Can you work these out from the model? Positions are in its coordinate system, mm. A direction names the side the tool comes from. Give positions to 0.01 mm unless a question says otherwise; leave off trailing zeros. Loops run counter-clockwise (first coordinate to the right, second up) from the corner with the lowest first, then second, coordinate; pieces in that order, holes last. Notation, with made-up numbers: (69.25, 76.25) - (96.25, 76.25) arc R35 cw to (96.25, 113.25) - close; hole circle Ø3 at (70, 32). An arc over 180 degrees is marked (long way). Answer as a JSON object with one key per item and string values. Group by question number.
Item 1: Suppose I cut it at B-B on z = 734.5. Write out the boundary of the cut face in (x, y), and give its area (3 significant figures).
Item 2: Suppose I cut it at C-C on x = -270. Write out the boundary of the cut face in (y, z), and give its area (3 significant figures).
Item 3: Suppose I cut it at D-D on x = -35. Write out the boundary of the cut face in (y, z), and give its area (3 significant figures).
Item 4: Suppose I cut it at A-A on y = 309.5. Write out the boundary of the cut face in (x, z).
Item 5: Which directions (+Z, -Z, +X, -X, +Y, -Y) give clear straight access to the entire face, cutting with the end or side of a thin tool? Please do faces 1 (the flat face through (-19, 461, 1160)), 2 (the flat face through (-7, 520, 1158.4)), 3 (the flat face through (-105.32, 697.036, 1159.211)).
Item 6: Will these pins go through, and if not, where does the flat tip stop? pin 1 (0.8 mm diameter, centred on x = -33.5, z = 0.5, fed in from +Y); pin 2 (10 mm diameter, centred on x = -288.5, z = 500.5, fed in from -Y); pin 3 (1.8 mm diameter, centred on x = 0.5, z = 512, fed in from +Y).
Item 7: Thinking about a two-plate mould opening in Y: for faces 4 (the flat face through (1.6, 236, 572)), 5 (the flat face through (-7, 517, 1.6)), 6 (the flat face through (-262, 801.6, 572)), 7 (the flat face through (-25, 0, 572)), which applies, pulls with the +Y half, pulls with the -Y half, needs draft (parallel to the pull), parting line crosses it, or undercut?
Item 8: Please list where these lines run through material, in increasing order: L1, parallel to Z at x = -15, y = 622; L2, parallel to Y at x = -251, z = 136; L3, parallel to X at y = 584, z = 485.
Autodesk Inventor part; units mm, degrees
ref_plane "YZ Plane" through (0, 0, 0) normal (1, 0, 0) x (0, 1, 0)
ref_plane "XZ Plane" through (0, 0, 0) normal (0, 1, 0) x (-1, 0, 0)
ref_plane "XY Plane" through (0, 0, 0) normal (0, 0, 1) x (1, 0, 0)
sketch "Sketch1" plane through (0, 0, 0) normal (0, 0, 1) x (1, 0, 0)
  line L0 (-347.6, 800) -> (-180, 800)
  line L1 (-180, 800) -> (0, 620)
  line L2 (-180, 800) -> (122.4624, 800) construction
  line L3 (0, 0) -> (0, 620)
  line L4 (0, 0) -> (-50, 0)
  line L5 (-50, -1.6) -> (1.6, -1.6)
  line L6 (1.6, -1.6) -> (1.6, 620.6627)
  line L7 (1.6, 620.6627) -> (-179.3373, 801.6)
  line L8 (-179.3373, 801.6) -> (-347.6, 801.6)
  line L9 (-347.6, 801.6) -> (-347.6, 800)
  line L10 (-50, 0) -> (-50, -1.6)
  dimension "d0" = 167.6
  dimension "d1" = 45
  dimension "d2" = 800
  dimension "d4" = 50
  dimension "d15" = 180
  dimension "d19" = 1.6
extrude "Extrusion1" add sketch "Sketch1" along normal blind 1160
sketch "Sketch2" plane through (0, 0, 0) normal (-1, 0, 0) x (0, 0, -1)
  line L0 (-195, -320) -> (-845, -320) construction
  line L1 (-845, -245) -> (-195, -245)
  line L2 (-195, -245) -> (-195, -395)
  line L3 (-195, -395) -> (-845, -395)
  line L4 (-845, -395) -> (-845, -245)
  point P0 (0, 0)
  dimension "d8" = 195
  dimension "d10" = 650
  dimension "d11" = 650
  dimension "d12" = 150
  dimension "d20" = 320
extrude "Extrusion3" cut sketch "Sketch2" against normal through all
sketch "Sketch3" plane through (0, 0, 0) normal (0, 0, -1) x (-1, 0, 0)
  line L0 (50, 0) -> (0, 0)
  line L1 (0, 0) -> (0, 620)
  line L2 (0, 620) -> (180, 800)
  line L3 (180, 800) -> (347.6, 800)
  line L4 (347.6, 780) -> (188.2843, 780)
  line L5 (188.2843, 780) -> (20, 611.7157)
  line L6 (20, 611.7157) -> (20, 20)
  line L7 (20, 20) -> (50, 20)
  line L8 (347.6, 780) -> (347.6, 800)
  line L9 (50, 20) -> (50, 0)
  dimension "d23" = 20
extrude "Extrusion4" add sketch "Sketch3" against normal blind 1.6
sketch "Sketch4" plane through (0, 0, 1160) normal (0, 0, 1) x (1, 0, 0)
  line L0 (0, 0) -> (-50, 0)
  line L1 (0, 620) -> (0, 0)
  line L2 (-180, 800) -> (0, 620)
  line L3 (-347.6, 800) -> (-180, 800)
  line L4 (-347.6, 800) -> (-347.6, 780)
  line L5 (-347.6, 780) -> (-188.2843, 780)
  line L6 (-188.2843, 780) -> (-20, 611.7157)
  line L7 (-20, 611.7157) -> (-20, 20)
  line L8 (-20, 20) -> (-50, 20)
  line L9 (-50, 20) -> (-50, 0)
extrude "Extrusion5" add sketch "Sketch4" against normal blind 1.6
sketch "Sketch5" plane through (-347.6, 801.6, 0) normal (-1, 0, 0) x (0, 0, 1)
  line L0 (1.6, -1.6) -> (1.6, -21.6)
  line L1 (1.6, -1.6) -> (1158.4, -1.6)
  line L2 (1158.4, -21.6) -> (1158.4, -1.6)
  line L3 (1.6, -21.6) -> (1158.4, -21.6)
  line L4 (0, 0) -> (0, -180.9373)
  point P0 (0, -801.6)
extrude "Extrusion6" add sketch "Sketch5" against normal blind 1.6
sketch "Sketch6" plane through (-347.6, 801.6, 0) normal (-1, 0, 0) x (0, 0, 1)
  line L0 (1158.4, -21.6) -> (1.6, -21.6)
  line L1 (580, -21.6) -> (580, 0) construction
  line L2 (0, 0) -> (1160, 0)
  line L3 (1.6, -1.6) -> (1158.4, -1.6)
  line L4 (1.6, -21.6) -> (1.6, -1.6)
  line L5 (3.2, -21.6) -> (3.2, -1.6)
  line L6 (1158.4, -1.6) -> (1158.4, -21.6)
  line L7 (1158.4, -181.6) -> (1158.4, -1.6)
  line L8 (1156.8, -1.6) -> (1156.8, -21.6)
  point P0 (0, -801.6)
  dimension "d30" = 1.6
  dimension "d31" = 1.6
extrude "Extrusion7" cut sketch "Sketch6" against normal blind 1.6 contours L0 L8 L3 L6 | L0 L4 L3 L5
properties part number "Cover Back" material "Steel"
Worked out:
{
 "1": {"outline": "(-347.6, 780) - (-346, 780) - (-346, 800) - (-180, 800) - (0, 620) - (0, 395) - (1.6, 395) - (1.6, 620.66) - (-179.34, 801.6) - (-347.6, 801.6) - close; (-50, -1.6) - (1.6, -1.6) - (1.6, 245) - (0, 245) - (0, 0) - (-50, 0) - close", "area": "1,540 mm2"},
 "2": {"outline": "(780, 0) - (801.6, 0) - (801.6, 1160) - (780, 1160) - (780, 1158.4) - (800, 1158.4) - (800, 1.6) - (780, 1.6) - close", "area": "1,920 mm2"},
 "3": {"outline": "(-1.6, 0) - (20, 0) - (20, 1.6) - (0, 1.6) - (0, 1158.4) - (20, 1158.4) - (20, 1160) - (-1.6, 1160) - close; (626.72, 0) - (657.26, 0) - (657.26, 1160) - (626.72, 1160) - (626.72, 1158.4) - (655, 1158.4) - (655, 1.6) - (626.72, 1.6) - close", "area": "4,640 mm2"},
 "4": {"outline": "(-20, 0) - (1.6, 0) - (1.6, 195) - (0, 195) - (0, 1.6) - (-20, 1.6) - close; (-20, 1158.4) - (0, 1158.4) - (0, 845) - (1.6, 845) - (1.6, 1160) - (-20, 1160) - close"},
 "5": {"face 1": "+Z, +X, -X, +Y, -Y", "face 2": "-X", "face 3": "+Z, -Z, -X"},
 "6": {"pin 1": "stops at y = 656.16", "pin 2": "stops at y = 800", "pin 3": "stops at y = 622.66"},
 "7": {"face 4": "needs draft", "face 5": "undercut", "face 6": "pulls with the +Y half", "face 7": "undercut"},
 "8": {"L1": "z = 0 to 1.6, 1158.4 to 1160", "L2": "y = 800 to 801.6", "L3": "x = 0 to 1.6"}
}
